Build history of the part. All positions in model axes, mm. A direction names the side the tool comes from. Give positions to 0.01 mm unless a question says otherwise; leave off trailing zeros. Loops run counter-clockwise (first coordinate to the right, second up) from the corner with the lowest first, then second, coordinate; pieces in that order, holes last. Notation, with made-up numbers: (-6.5, -40) - (2.5, -40) arc R28 ccw to (2.5, -7) - close; hole circle Ø6 at (81.5, 1). An arc over 180 degrees is marked (long way). Return JSON: item names as keys, results as strings. Group by question number.
1) Slice it at C-C (y = 15). List the corners of the cut face in (x, z).
2) Mould opens along Z. For faces 1 (the face through (0, 75, 41)), 2 (the face through (-13, 75, 152.4)), 3 (the face through (-12.52, 66.72, 143.62)) say: released by +Z, released by -Z, zero draft, split by the parting line, or undercut.
3) Slice it at B-B (z = 103). List the corners of the cut face in (x, y), and give its area (3 significant figures).
4) Slice it at D-D (x = -10.5). List the corners of the cut face in (y, z), and give its area (3 significant figures).
5) Slice it at A-A (y = 43). List the corners of the cut face in (x, z).
6) Drop a flat-ended pin along its axis: pin 1 (5 mm diameter, centred on x = -30.5, y = 71, fed in from +Z). Give the stop position or say it passes through.
7) 3-axis set-ups, long thin cutter, end or side, ignore diameter. For faces 4 (the face through (-25.4, 75, 47)), 5 (the face through (-22, 152.4, 60)): which of +Z, -Z, +X, -X, +Y, -Y reach the whole face in a straight line?
8) Drill centre lines: probe 1 along X at (y, z) = (107.5, 38.5); probe 2 along Z at (x, y) = (-64.5, 19); probe 3 along Z at (x, y) = (-5.5, 94). Where is each one in solid material? Low to high. Write a range as from..to.
```python
from build123d import *

# Parameters (mm, degrees)
F1_DEPTH = 152.4
F2_R     = 47.9646820368
F3_DEPTH = 152.4


# Not quite as in the source:
# - a feature names something its author has since deleted; it is built from what else it names


with BuildPart() as f1:
    # F0 (on Front) → F1 (new body)
    with BuildSketch(Plane.XZ):
        Polygon((-76.2, 0), (0, 0), (0, 152.4), (-25.4, 152.4), (-25.4, 25.4), (-76.2, 25.4), align=None)
    extrude(amount=-F1_DEPTH)

    # F2 (on Right) → F3 (cut)
    with BuildSketch(Plane.YZ):
        with Locations((72.9622766376, 96.0644483566)):
            Circle(F2_R)
    extrude(amount=-F3_DEPTH, mode=Mode.SUBTRACT)


solid = f1.part
```
Results:
{
 "1": {"outline": "(-76.2, 0) - (0, 0) - (0, 152.4) - (-25.4, 152.4) - (-25.4, 25.4) - (-76.2, 25.4) - close"},
 "2": {"face 1": "zero draft", "face 2": "released by +Z", "face 3": "undercut"},
 "3": {"outline": "(-25.4, 0) - (0, 0) - (0, 25.5) - (-25.4, 25.5) - close; (-25.4, 120.42) - (0, 120.42) - (0, 152.4) - (-25.4, 152.4) - close", "area": "1,460 mm2"},
 "4": {"outline": "(0, 0) - (152.4, 0) - (152.4, 152.4) - (0, 152.4) - close; hole circle Ø95.93 at (72.96, 96.06)", "area": "16,000 mm2"},
 "5": {"outline": "(-76.2, 0) - (0, 0) - (0, 58.61) - (-25.4, 58.61) - (-25.4, 25.4) - (-76.2, 25.4) - close; (-25.4, 133.52) - (0, 133.52) - (0, 152.4) - (-25.4, 152.4) - close"},
 "6": {"pin 1": "z = 25.4"},
 "7": {"face 4": "+Z, -X, +Y, -Y", "face 5": "+Z, -Z, +X, -X, +Y"},
 "8": {"probe 1": "-25.4..0", "probe 2": "0..25.4", "probe 3": "0..52.96, 139.17..152.4"}
}
